```python
from build123d import *

# Parameters (mm, degrees)
BINDER_R        = 1.62
PAD_DEPTH       = 2
SKETCH_R        = 1.68
POCKET_DEPTH    = 2
SKETCH001_R     = 2.5
PAD001_DEPTH    = 0.5
SKETCH002_R     = 1.64
POCKET001_DEPTH = 2.5


with BuildPart() as part:
    # Binder → Pad (new body)
    with BuildSketch(Plane(origin=(-2.505049, -4.237344, 0), x_dir=(0, 1, 0), z_dir=(0, 0, 1))):
        with BuildLine():
            ThreePointArc((-8.205901, 3.106567), (-10.451974, 0.288635), (-8.371302, -2.653539))
            Line((-8.371302, -2.653539), (3.01322, -6.313136))
            ThreePointArc((3.01322, -6.313136), (6.59356, -5.737424), (8.237344, -2.505049))
            Line((8.237344, -2.505049), (8.237344, 5.294951))
            Line((8.237344, 5.294951), (0.237344, 5.294951))
            Line((0.237344, 5.294951), (-8.205901, 3.106567))
        make_face()
        with Locations((4.237344, -2.505049)):
            Circle(BINDER_R, mode=Mode.SUBTRACT)
    extrude(amount=-PAD_DEPTH)

    # Sketch (on Face9 of Pad) → Pocket (cut)
    with BuildSketch(Plane(origin=(0, 0, -2), x_dir=(1, 0, 0), z_dir=(0, 0, -1))):
        with Locations((-5, 0)):
            Circle(SKETCH_R)
    extrude(amount=-POCKET_DEPTH, mode=Mode.SUBTRACT)

    # Sketch001 (on Face5 of Pocket) → Pad001 (join)
    with BuildSketch(Plane(origin=(0, 0, -2), x_dir=(1, 0, 0), z_dir=(0, 0, -1))):
        with Locations((-2.707575, 11.690553)):
            Circle(SKETCH001_R)
    extrude(amount=PAD001_DEPTH)

    # Sketch002 (on Face12 of Pad001) → Pocket001 (cut)
    with BuildSketch(Plane(origin=(0, 0, -2.5), x_dir=(1, 0, 0), z_dir=(0, 0, -1))):
        with Locations((-2.707575, 11.690553)):
            Circle(SKETCH002_R)
    extrude(amount=-POCKET001_DEPTH, mode=Mode.SUBTRACT)


solid = part.part
```
Geometry: final body of the model. Coordinates: model frame, mm. Round coordinates to 2 decimals unless told otherwise and drop trailing zeros. Order: outer loops, then holes, each group sorted by start corner. A loop starts at its lowest first (then second) coordinate and runs counter-clockwise, first axis right, second up. Notation, with made-up numbers: M 23,64 L 55,64 A18 ccw 55,92 Z; hole C 69,54.25 d1. An arc over 180 degrees is marked long. Use one line per item in the form item = value. Start each with the question number.
Q1. Cut plane D-D (x = -3.5). Return loops of the section in (y, z), and give its area (3 significant figures).
Q2. Pin query (flat end, axial travel): pin 1 Ø2.5 at (x, y) = (-2.71, -11.69) entering from +Z. Return the tip coordinate at first contact, or that it passes through.
Q3. Cut plane A-A (x = -6.25). Return loops of the section in (y, z), and give its area (3 significant figures).
Q4. Material intervals for line 1 (X direction, y = 0, z = -0.5); line 2 (Y direction, x = -3.5, z = -0.8); line 3 (Y direction, x = -3.75, z = -0.65), sorted ascending. Write a range as [from, to].
Q5. Cut plane B-B (y = 0). Return loops of the section in (x, z).
Q6. Cut plane C-C (y = -12). Return loops of the section in (x, z), and give its area (3 significant figures).
Q7. Mould query, pull axis Y, two halves, no side actions, for faces 1 (the face through (-3.448, 0.643, -1.014)), 2 (the face through (-7.8, 0, -1)), 3 (the face through (-4.69, -10.17, -2.25)). Classes: +Y half, -Y half, draft (parallel to the pull), parting line (faces both ways), or undercut.
Geometry results:
q1.outline = M -14.58,-2 L -14.06,-2 L -14.06,-2.5 L -13.13,-2.5 L -13.13,0 L -14.58,0 Z; M -10.25,-2.5 L -9.32,-2.5 L -9.32,-2 L -0.76,-2 L -0.76,0 L -10.25,0 Z; M 0.76,-2 L 4,-2 L 4,0 L 0.76,0 Z
q1.area = 29.3 mm^2
q2.pin_1 = through
q3.outline = M -9.98,-2 L -1.12,-2 L -1.12,0 L -9.98,0 Z; M 1.12,-2 L 4,-2 L 4,0 L 1.12,0 Z
q3.area = 23.5 mm^2
q4.line_1 = [-7.8, -6.68], [-3.32, -1.62], [1.62, 4]
q4.line_2 = [-14.58, -13.13], [-10.25, -0.76], [0.76, 4]
q4.line_3 = [-14.5, -12.96], [-10.42, -1.12], [1.12, 4]
q5.outline = M -7.8,-2 L -6.68,-2 L -6.68,0 L -7.8,0 Z; M -3.32,-2 L -1.62,-2 L -1.62,0 L -3.32,0 Z; M 1.62,-2 L 4,-2 L 4,0 L 1.62,0 Z
q6.outline = M -5.73,-2 L -5.19,-2 L -5.19,-2.5 L -4.32,-2.5 L -4.32,0 L -5.73,0 Z; M -1.1,-2.5 L -0.23,-2.5 L -0.23,-2 L 0.34,-2 L 0.34,0 L -1.1,0 Z
q6.area = 6.57 mm^2
q7.face_1 = undercut
q7.face_2 = draft
q7.face_3 = parting line
